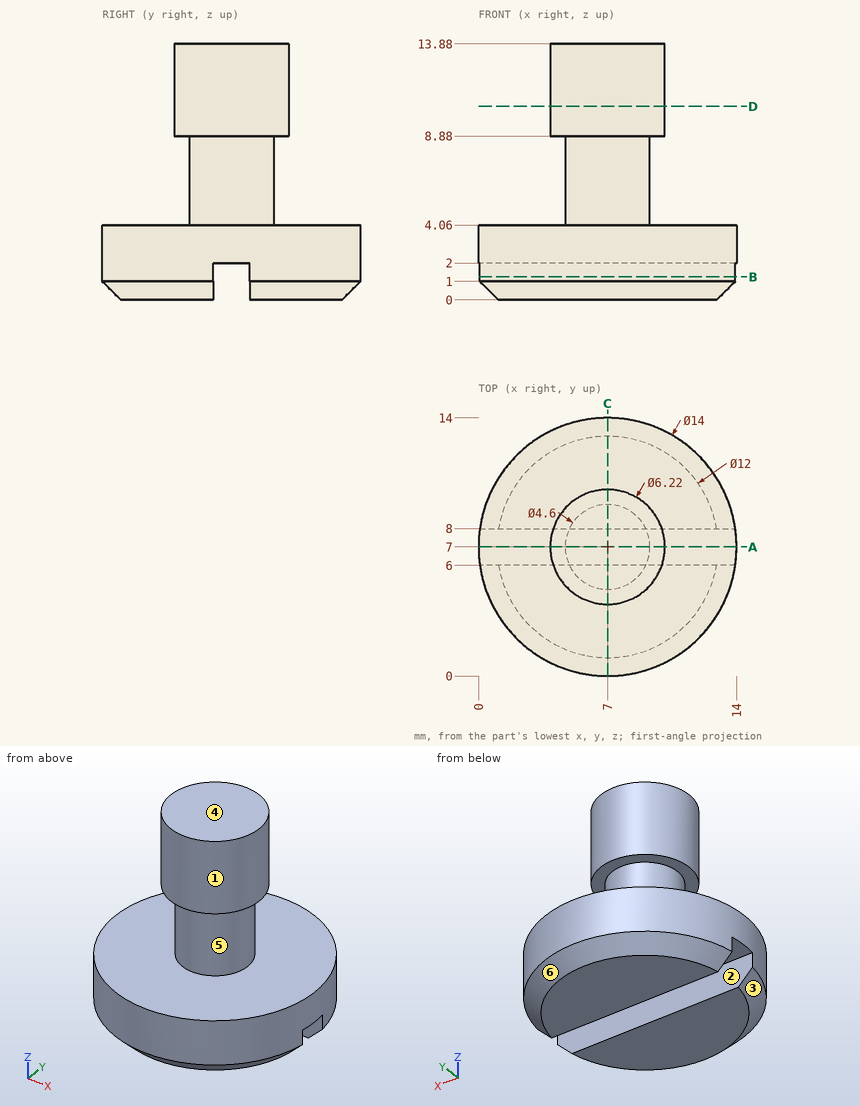
Print and shaded views of the part. All mm, measured from the part's lowest x, y and z. A direction names the side the tool comes from. Coordinates: 2 decimals unless noted, no trailing zeros. Loops run counter-clockwise (first coordinate to the right, second up) from the corner with the lowest first, then second, coordinate; pieces in that order, holes last. Notation, with made-up numbers: (-27.5, -16) - (-16.5, -16) arc R18 cw to (-16.5, -9) - close; hole circle Ø11 at (-14.5, 21.25). An arc over 180 degrees is marked (long way). Write item = value, one per line. Start each with the question number.
Item 1: 3-axis set-ups, long thin cutter, end or side, ignore diameter. For the marked faces 1, 2 and 3: which of +Z, -Z, +X, -X, +Y, -Y reach the whole face in a straight line?
Item 2: Saw through at B-B, the plane z = 1.25. List the corners of the cut face in (x, y).
Item 3: Saw through at A-A, the plane y = 7. List the corners of the cut face in (x, z), then the cut area to 3 significant figures.
Item 4: Saw through at C-C, the plane x = 7. List the corners of the cut face in (y, z), then the cut area to 3 significant figures.
Item 5: Pull direction Z, two halves, no side cores. Call the marked faces 4, 5 and 6: +Z half, -Z half, draft (parallel to the pull), parting line (faces both ways), or undercut.
Item 6: Wall check: probe 1 along Z at (x, y) = (5.5, 3.5); probe 2 along Z at (x, y) = (9, 7.5); probe 3 along Y at (x, z) = (8, 13). Give the ranges that are in metal, low to high. Write a range as [from, to].
Item 7: Saw through at D-D, the plane z = 10.5. List the corners of the cut face in (x, y).
Item 8: Drop flat-ended pins along their axis: pin 1 Ø2 at (x, y) = (2.5, 4) entering from -Z; pin 2 Ø0.6 at (x, z) = (9, 1) entering from -Y; pin 3 Ø1.5 at (y, z) = (9, 8) entering from +X; pin 4 Ø1.6 at (x, y) = (5, 7) entering from -Z. Give the stop position or say it passes through.
Answers:
q1.face_1 = +Z
q1.face_2 = -Z, +X, -X
q1.face_3 = -Z, -Y
q2.outline = (0.07, 6) arc R7 ccw to (13.93, 6) - close; (0.07, 8) - (13.93, 8) arc R7 ccw to start
q3.outline = (0, 2) - (14, 2) - (14, 4.06) - (9.3, 4.06) - (9.3, 8.88) - (10.11, 8.88) - (10.11, 13.88) - (3.89, 13.88) - (3.89, 8.88) - (4.7, 8.88) - (4.7, 4.06) - (0, 4.06) - close
q3.area = 82.1 mm2
q4.outline = (0, 1) - (1, 0) - (6, 0) - (6, 2) - (8, 2) - (8, 0) - (13, 0) - (14, 1) - (14, 4.06) - (9.3, 4.06) - (9.3, 8.88) - (10.11, 8.88) - (10.11, 13.88) - (3.89, 13.88) - (3.89, 8.88) - (4.7, 8.88) - (4.7, 4.06) - (0, 4.06) - close
q4.area = 105 mm2
q5.face_4 = +Z half
q5.face_5 = undercut
q5.face_6 = -Z half
q6.probe_1 = [0, 4.06]
q6.probe_2 = [2, 13.88]
q6.probe_3 = [4.06, 9.94]
q7.outline = circle Ø6.22 at (7, 7)
q8.pin_1 = 0
q8.pin_2 = 0.21
q8.pin_3 = 8.93
q8.pin_4 = 2
